from build123d import *

# Parameters (mm, degrees)
EXTRUDE_1_DEPTH     = 40.5
SKETCH_2_W          = 4.25
SKETCH_2_H          = 6
SKETCH_2_R          = 1
EXTRUDE_2_DEPTH     = 19
EXTRUDE_START       = 6.9
SKETCH_6_W          = 3
SKETCH_6_H          = 12
SKETCH_6_R          = 1
EXTRUDE_3_DEPTH     = 6.9
SKETCH_7_W          = 10
SKETCH_7_H          = 3
CUT_EXTRUDE_1_DEPTH = 4
SKETCH_9_R          = 2
CUT_EXTRUDE_2_DEPTH = 2
SKETCH_10_R         = 1
CUT_EXTRUDE_3_DEPTH = 12
SKETCH_12_W         = 0.5
SKETCH_12_H         = 19
CUT_EXTRUDE_4_DEPTH = 0.5


with BuildPart() as part:
    # 草图1 → 凸台-拉伸1 (new body)
    with BuildSketch(Plane.XY):
        Polygon((3, -13), (-5, -13), (-5, -7), (0, -7), (0, 0), (-5, 0), (-5, 6), (3, 6), align=None)
    extrude(amount=EXTRUDE_1_DEPTH)

    # 草图2 → 凸台-拉伸2 (add)
    with BuildSketch(Plane(origin=(0, 6, 0), x_dir=(1, 0, 0), z_dir=(0, 1, 0))):
        with Locations((5.125, -8)):
            Rectangle(SKETCH_2_W, SKETCH_2_H)
        with Locations(Location((4.25, -8, 0), (0, 0, 270))):
            Circle(SKETCH_2_R, mode=Mode.SUBTRACT)
    extrude(amount=-EXTRUDE_2_DEPTH)

    # 草图6 → 凸台-拉伸3 (add)
    # profile 1 of 2: a face of its own
    with BuildSketch(Plane(origin=(0, 6, 0), x_dir=(1, 0, 0), z_dir=(0, 1, 0)).offset(EXTRUDE_START)):
        with Locations((1.5, -34.5)):
            Rectangle(SKETCH_6_W, SKETCH_6_H)
    # profile 2 of 2: a face of its own
    with BuildSketch(Plane(origin=(0, 6, 0), x_dir=(1, 0, 0), z_dir=(0, 1, 0)).offset(EXTRUDE_START)):
        with BuildLine():
            Line((4.25, -10.5), (3, -10.5))
            Line((3, -10.5), (3, -12))
            Line((3, -12), (0, -12))
            Line((0, -12), (0, 0))
            Line((0, 0), (3, 0))
            Line((3, 0), (3, -5.5))
            Line((3, -5.5), (4.25, -5.5))
            ThreePointArc((4.25, -5.5), (6.75, -8), (4.25, -10.5))
        make_face()
        with Locations(Location((4.25, -8, 0), (0, 0, 270))):
            Circle(SKETCH_6_R, mode=Mode.SUBTRACT)
    extrude(amount=-EXTRUDE_3_DEPTH)

    # 草图7 → 切除-拉伸1 (cut)
    with BuildSketch(Plane(origin=(3, 0, 0), x_dir=(0, 0, -1), z_dir=(1, 0, 0))):
        with Locations((-20.25, -11.5)):
            Rectangle(SKETCH_7_W, SKETCH_7_H)
    extrude(amount=-CUT_EXTRUDE_1_DEPTH, mode=Mode.SUBTRACT)

    # 草图9 → 切除-拉伸2 (cut)
    with BuildSketch(Plane.ZY.offset(5)):
        with Locations((37.5, -10)):
            Circle(SKETCH_9_R)
        with Locations((3, -10)):
            Circle(SKETCH_9_R)
    extrude(amount=-CUT_EXTRUDE_2_DEPTH, mode=Mode.SUBTRACT)

    # 草图10 → 切除-拉伸3 (cut)
    with BuildSketch(Plane.ZY.offset(3)):
        with Locations((37.5, -10)):
            Circle(SKETCH_10_R)
        with Locations((3, -10)):
            Circle(SKETCH_10_R)
    extrude(amount=-CUT_EXTRUDE_3_DEPTH, mode=Mode.SUBTRACT)

    # 草图12 → 切除-拉伸4 (cut)
    with BuildSketch(Plane.ZY.offset(5)):
        with Locations((12.25, -3.5)):
            Rectangle(SKETCH_12_W, SKETCH_12_H)
        with Locations((28.25, -3.5)):
            Rectangle(SKETCH_12_W, SKETCH_12_H)
    extrude(amount=-CUT_EXTRUDE_4_DEPTH, mode=Mode.SUBTRACT)


solid = part.part
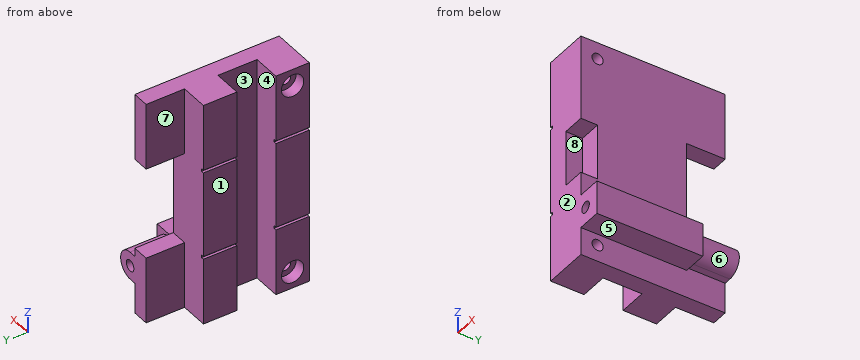
CAD build for the part. Positions are in the model's coordinates, mm. Face numbers are marked on the shaded views. A direction names the side the tool comes from. Give positions to 0.01 mm unless a question says otherwise; leave off trailing zeros. Loops run counter-clockwise (first coordinate to the right, second up) from the corner with the lowest first, then second, coordinate; pieces in that order, holes last. Notation, with made-up numbers: M 68,38.5 L 85,38.5 A21 cw 85,50.5 Z; hole C -11,43 d10. An arc over 180 degrees is marked long. One line per question, with ' | ' between items. Start each with the question number.
1. Saw through at C-C on y = -3.5. Give the cut face in (x, z).
2. Saw through at A-A on y = 10.5. Give the cut face in (x, z).
3. Probe L1, parallel to Y at x = -3.8, z = 3; L2, parallel to Z at x = 1.75, y = 8.25; L3, parallel to Y at x = -0.75, z = 3. List the from-to ranges inside material, lowest first. Write a range as from..to.
4. Saw through at B-B on z = 3. Give the cut face in (x, y), plus the area to 3 significant figures.
5. 3-axis set-ups, long thin cutter, end or side, ignore diameter. For the marked faces 5, 6, 7 and 8: which of +Z, -Z, +X, -X, +Y, -Y reach the whole face in a straight line?
6. Flat gauge pins, fed straight in: pin 1 (1.2 mm diameter, centred on x = 1, z = 21, fed in from -Y); pin 2 (4.5 mm diameter, centred on x = 5, z = 8.5, fed in from +Y); pin 3 (4 mm diameter, centred on x = -2, z = 15.5, fed in from +Y); pin 4 (12 mm diameter, centred on y = 2, z = 27.5, fed in from +X). Where does each tip first touch, or does it go through?
7. Saw through at D-D on z = 9.5. Give the cut face in (x, y).
8. Two-plate mould, pull along Y, no slides. Class the marked faces 1, 2, 3 and 4: pulls with the +Y half, pulls with the -Y half, needs draft (parallel to the pull), parting line crosses it, or undercut.
Result sheet:
1) outline: M 0,0 L 3,0 L 3,5 L 7.25,5 L 7.25,11 L 3,11 L 3,40.5 L 0,40.5 Z; hole C 4.25,8 d2
2) outline: M 0,0 L 3,0 L 3,5.5 L 4.25,5.5 A2.5 ccw 4.25,10.5 L 3,10.5 L 3,12 L 0,12 Z; M 0,28.5 L 3,28.5 L 3,40.5 L 0,40.5 Z; hole C 4.25,8 d2
3) L1: y = -13..-12, -8..-7, 0..6 | L2: z = 0..12, 28.5..40.5 | L3: y = -13..-11, -9..-7, 0..6
4) outline: M -5,-13 L 3,-13 L 3,-11 L -3,-11 L -3,-12 L -5,-12 Z; M -5,-8 L -3,-8 L -3,-9 L 3,-9 L 3,12.9 L 0,12.9 L 0,6 L -5,6 L -5,0 L 0,0 L 0,-7 L -5,-7 Z | area: 118 mm^2
5) face 5: -Z, +X, +Y, -Y | face 6: +X, +Y | face 7: +Z, -Z, -X, +Y | face 8: +X, -Y
6) pin 1: stops at y = -10 | pin 2: stops at y = 12.9 | pin 3: stops at y = 6 | pin 4: stops at x = 3
7) outline: M -5,-13 L 7.25,-13 L 7.25,6 L 6.25,6 L 6.25,12.9 L 0,12.9 L 0,6 L -5,6 L -5,0 L 0,0 L 0,-7 L -5,-7 Z
8) face 1: needs draft | face 2: pulls with the -Y half | face 3: undercut | face 4: undercut
